from build123d import *

# Parameters (mm, degrees)
BOSS_EXTRUDE1_DEPTH     = 38
CUT_EXTRUDE1_REACH      = 43.037
SKETCH2_R               = 2.15
CUT_EXTRUDE4_DEPTH      = 42.036691991
CUT_EXTRUDE4_DEPTH_BACK = 42.036691991
SKETCH3_W               = 10
SKETCH3_H               = 1
SKETCH3_H_2             = 4.881241343


with BuildPart() as part:
    # Sketch1 → Boss-Extrude1 (new body)
    with BuildSketch(Plane.XY):
        with BuildLine():
            Line((0.8, -0.368758657), (0.8, 15.131241343))
            Line((0.8, 15.131241343), (0, 15.131241343))
            Line((0, 15.131241343), (0, 0))
            ThreePointArc((0, 0), (-0.08085497, -0.393919299), (-0.310344828, -0.724137931))
            ThreePointArc((-0.310344828, -0.724137931), (2.474900525, -5.062251314), (1.5, 0))
            Line((1.5, 0), (1.5, -0.8))
            ThreePointArc((1.5, -0.8), (2.079032119, -4.355707025), (0.401769912, -1.167428159))
            ThreePointArc((0.401769912, -1.167428159), (0.69492176, -0.814981745), (0.8, -0.368758657))
        make_face()
    extrude(amount=BOSS_EXTRUDE1_DEPTH)

    # Sketch2 → Cut-Extrude1 (cut, up to next)
    with BuildSketch(Plane(origin=(0.8, 0, 0), x_dir=(0, 0, -1), z_dir=(1, 0, 0)), mode=Mode.PRIVATE) as cut_extrude1_sk1:
        with Locations((-30.5, 7.381241343)):
            Circle(SKETCH2_R)
    cut_extrude1_tool1 = extrude(cut_extrude1_sk1.sketch, amount=-CUT_EXTRUDE1_REACH, mode=Mode.PRIVATE) & part.part
    # Sketch2 → Cut-Extrude1 (cut, up to next)
    with BuildSketch(Plane(origin=(0.8, 0, 0), x_dir=(0, 0, -1), z_dir=(1, 0, 0)), mode=Mode.PRIVATE) as cut_extrude1_sk2:
        with Locations((-7.5, 7.381241343)):
            Circle(SKETCH2_R)
    cut_extrude1_tool2 = extrude(cut_extrude1_sk2.sketch, amount=-CUT_EXTRUDE1_REACH, mode=Mode.PRIVATE) & part.part
    add(cut_extrude1_tool1.solids().sort_by_distance((0.8, 7.381241, 30.5))[0], mode=Mode.SUBTRACT)
    add(cut_extrude1_tool2.solids().sort_by_distance((0.8, 7.381241, 7.5))[0], mode=Mode.SUBTRACT)

    # Sketch3 → Cut-Extrude4 (cut, two sides: drawn at the far end of the back side and taken through both)
    with BuildSketch(Plane(origin=(0.8, 0, 0), x_dir=(0, 0, -1), z_dir=(1, 0, 0)).offset(-CUT_EXTRUDE4_DEPTH_BACK)):
        with Locations((-33, 0.131241343)):
            Rectangle(SKETCH3_W, SKETCH3_H)
        with Locations((-33, -2.809379328)):
            Rectangle(SKETCH3_W, SKETCH3_H_2)
        with Locations((-5, 0.131241343)):
            Rectangle(SKETCH3_W, SKETCH3_H)
        with Locations((-5, -2.809379328)):
            Rectangle(SKETCH3_W, SKETCH3_H_2)
    extrude(amount=CUT_EXTRUDE4_DEPTH + CUT_EXTRUDE4_DEPTH_BACK, mode=Mode.SUBTRACT)


solid = part.part
Model file for the job. Use its own axes, mm. A direction names the side the tool comes from. Coordinates: 2 decimals unless noted, no trailing zeros. Write each loop counter-clockwise with the first axis right and the second up, starting at its lowest first coordinate (ties: lowest second). Pieces come first, ordered by that corner, then holes. Notation, with made-up numbers: (-25.75, -6) -> (-0.75, -6) arc R21 cw to (-0.75, 9) -> close; hole circle Ø2 at (2.5, 55.25). An arc over 180 degrees is marked (long way). One line per item, written item: value. Start each with the question number.
1) Probe probe 1 along Y at (x, z) = (0.4, 30.5); probe 2 along X at (y, z) = (5, 24.5); probe 3 along Z at (x, y) = (3.4, -2.5). List the from-to ranges inside material, lowest first.
2) Flat gauge pins, fed straight in: pin 1 Ø5.5 at (y, z) = (7.38, 30.5) entering from -X; pin 2 Ø0.9 at (y, z) = (-0.5, 18.5) entering from -X; pin 3 Ø2 at (y, z) = (9, 15.5) entering from +X; pin 4 Ø3 at (x, z) = (2.5, 6.5) entering from -Y. Where does each tip first touch, or does it go through?
3) Which spindle directions (+Z, -Z, +X, -X, +Y, -Y) get a long thin tool onto all of the face, cutting with end or side? Do faces 4 (the face through (0, -4, 28)), 5 (the face through (1.5, -0.4, 18.9)), 6 (the face through (0, 8, 19)). Say none if no direction does.
4) Slice it at B-B on y = 8. Write the cut outline in (x, z), then the cut area to 3 significant figures.
5) Slice it at A-A on z = 7.5. Write the cut outline in (x, y).
6) Slice it at C-C on x = 2.25. Write the cut outline in (y, z).
7) Pull direction Z, two halves, no side cores. Call faces 1 (the face through (0, -4, 10)), 2 (the face through (2.38, -5.1, 18.87)), 3 (the face through (0.41, 8.03, 5.45)): +Z half, -Z half, draft (parallel to the pull), parting line (faces both ways), or undercut.
8) Slice it at D-D on z = 23. Write the cut outline in (x, y) (3 decimals).
Answers follow:
1. probe 1: 0.63 to 5.23, 9.53 to 15.13
1. probe 2: 0 to 0.8
1. probe 3: 10 to 28
2. pin 1: x = 0
2. pin 2: x = -0.52
2. pin 3: x = 0.8
2. pin 4: through
3. face 4: +Z, +X, -X, -Y
3. face 5: +Z, -Z, +Y
3. face 6: +Z, -Z, -X, +Y
4. outline: (0, 0) -> (0.8, 0) -> (0.8, 5.44) -> (0, 5.44) -> close; (0, 9.56) -> (0.8, 9.56) -> (0.8, 28.44) -> (0, 28.44) -> close; (0, 32.56) -> (0.8, 32.56) -> (0.8, 38) -> (0, 38) -> close
4. area: 23.8 mm2
5. outline: (0, 0.63) -> (0.8, 0.63) -> (0.8, 5.23) -> (0, 5.23) -> close; (0, 9.53) -> (0.8, 9.53) -> (0.8, 15.13) -> (0, 15.13) -> close
6. outline: (-5.14, 10) -> (-4.29, 10) -> (-4.29, 28) -> (-5.14, 28) -> close; (-0.96, 10) -> (-0.11, 10) -> (-0.11, 28) -> (-0.96, 28) -> close
7. face 1: -Z half
7. face 2: draft
7. face 3: undercut
8. outline: (-0.31, -0.724) arc R2.625 ccw (long way) to (1.5, 0) -> (1.5, -0.8) arc R1.825 cw (long way) to (0.402, -1.167) arc R1 ccw to (0.8, -0.369) -> (0.8, 15.131) -> (0, 15.131) -> (0, 0) arc R1 cw to start
